Could you check a few things on this model? Use its own coordinates, in mm. Give positions to 0.01 mm unless a question says otherwise; leave off trailing zeros. Order: outer loops, then holes, each group sorted by start corner. A loop starts at its lowest first (then second) coordinate and runs counter-clockwise, first axis right, second up. Notation, with made-up numbers: M 56,69.25 L 110,69.25 A17 ccw 110,84.25 Z; hole C -36.75,25.5 d10. An arc over 180 degrees is marked long. Answer in a Markdown table with one row per item. Add a question column.
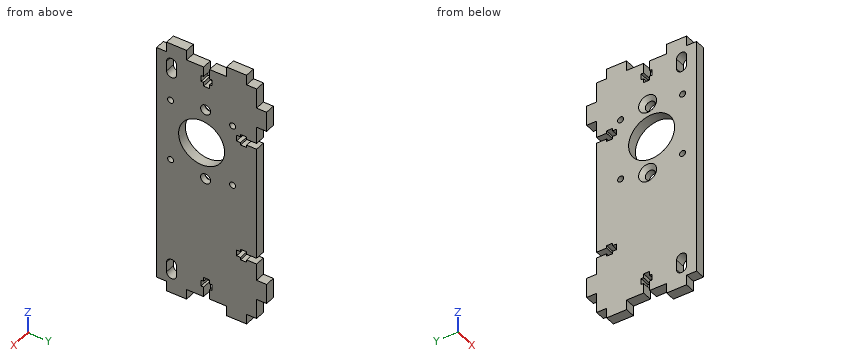
```python
from build123d import *

# Parameters (mm, degrees)
SKETCH1_W           = 120
SKETCH1_H           = 50
SKETCH1_R           = 1.5
SKETCH1_R_2         = 11.5
SKETCH1_R_3         = 2.5
BOSS_EXTRUDE1_DEPTH = 5
CHAMFER1_SIZE       = 2
SKETCH2_W           = 5
SKETCH2_H           = 10
SKETCH2_W_2         = 10
SKETCH2_H_2         = 5
BOSS_EXTRUDE2_DEPTH = 5
CUT_EXTRUDE1_DEPTH  = 137.656503687


with BuildPart() as part:
    # Sketch1 → Boss-Extrude1 (new body)
    with BuildSketch(Plane(origin=(0, 0, 0), x_dir=(0, 0, -1), z_dir=(1, 0, 0))):
        with Locations((-60, 25)):
            Rectangle(SKETCH1_W, SKETCH1_H)
        with Locations((-95.5, 38)):
            Circle(SKETCH1_R, mode=Mode.SUBTRACT)
        with Locations((-64.5, 38)):
            Circle(SKETCH1_R, mode=Mode.SUBTRACT)
        with Locations((-64.5, 7)):
            Circle(SKETCH1_R, mode=Mode.SUBTRACT)
        with Locations((-95.5, 7)):
            Circle(SKETCH1_R, mode=Mode.SUBTRACT)
        with Locations((-80, 22.5)):
            Circle(SKETCH1_R_2, mode=Mode.SUBTRACT)
        with Locations((-98, 24.5)):
            Circle(SKETCH1_R_3, mode=Mode.SUBTRACT)
        with Locations((-62, 24.5)):
            Circle(SKETCH1_R_3, mode=Mode.SUBTRACT)
    extrude(amount=BOSS_EXTRUDE1_DEPTH)

    # Chamfer1
    chamfer1_edges = [part.edges().sort_by_distance(p)[0] for p in [
        (0, 24.5, 100.5),
        (0, 24.5, 64.5),
    ]]
    chamfer(chamfer1_edges, length=CHAMFER1_SIZE)

    # Sketch2 → Boss-Extrude2 (add)
    with BuildSketch(Plane(origin=(5, 0, 0), x_dir=(0, 0, -1), z_dir=(1, 0, 0))):
        with Locations((-122.5, 10)):
            Rectangle(SKETCH2_W, SKETCH2_H)
        with Locations((-122.5, 40)):
            Rectangle(SKETCH2_W, SKETCH2_H)
        with Locations((-105, 52.5)):
            Rectangle(SKETCH2_W_2, SKETCH2_H_2)
        with Locations((-15, 52.5)):
            Rectangle(SKETCH2_W_2, SKETCH2_H_2)
        with Locations((2.5, 40)):
            Rectangle(SKETCH2_W, SKETCH2_H)
        with Locations((2.5, 10)):
            Rectangle(SKETCH2_W, SKETCH2_H)
    extrude(amount=-BOSS_EXTRUDE2_DEPTH)

    # Sketch3 → Cut-Extrude1 (cut, through all)
    with BuildSketch(Plane(origin=(5, 0, 0), x_dir=(0, 0, -1), z_dir=(1, 0, 0))):
        Polygon((0, 26.5), (-5, 26.5), (-5, 27.75), (-8, 27.75), (-8, 26.5), (-10, 26.5), (-10, 23.5), (-8, 23.5), (-8, 22.25), (-5, 22.25), (-5, 23.5), (0, 23.5), align=None)
        Polygon((-120, 23.5), (-120, 26.5), (-115, 26.5), (-115, 27.75), (-112, 27.75), (-112, 26.5), (-110, 26.5), (-110, 23.5), (-112, 23.5), (-112, 22.25), (-115, 22.25), (-115, 23.5), align=None)
        Polygon((-31.5, 50), (-31.5, 45), (-32.75, 45), (-32.75, 42), (-31.5, 42), (-31.5, 40), (-28.5, 40), (-28.5, 42), (-27.25, 42), (-27.25, 45), (-28.5, 45), (-28.5, 50), align=None)
        Polygon((-91.5, 50), (-88.5, 50), (-88.5, 45), (-87.25, 45), (-87.25, 42), (-88.5, 42), (-88.5, 40), (-91.5, 40), (-91.5, 42), (-92.75, 42), (-92.75, 45), (-91.5, 45), align=None)
        with BuildLine():
            Line((-115, 10), (-110, 10))
            ThreePointArc((-110, 10), (-107.5, 7.5), (-110, 5))
            Line((-110, 5), (-115, 5))
            ThreePointArc((-115, 5), (-117.5, 7.5), (-115, 10))
        make_face()
        with BuildLine():
            Line((-5, 10), (-10, 10))
            ThreePointArc((-10, 10), (-12.5, 7.5), (-10, 5))
            Line((-10, 5), (-5, 5))
            ThreePointArc((-5, 5), (-2.5, 7.5), (-5, 10))
        make_face()
    extrude(amount=-CUT_EXTRUDE1_DEPTH, mode=Mode.SUBTRACT)


solid = part.part
```
1. Suppose I cut it at C-C on y = 7. List the corners of the cut face in (x, z) for me, plus the area to 3 significant figures.
2. Will these pins go through, and if not, where does the flat tip stop? P1, Ø1.5, axis at x = 3.5, y = 32, coming from the +Z side; P2, Ø2.5, axis at x = 1.5, y = 53.5, coming from the +Z side; P3, Ø2.5, axis at x = 2, z = 117, coming from the +Y side.
3. Suppose I cut it at A-A on y = 38. List the corners of the cut face in (x, z) for me, plus the area to 3 significant figures.
4. If I drill on line 1 along Y through (x, z) = (3.2, 110.5); line 2 along Z through (x, y) = (1.3, 41.5); line 3 along Y through (x, z) = (3.5, 62), over which ranges is the centre line in solid material (lowest first)? Write a range as [from, to].
5. Suppose I cut it at D-D on x = 3.9. Count the separate pieces of the cut face and the enclosed holes in it, plus the area to 3 significant figures.
6. Suppose I cut it at B-B on y = 17. List the corners of the cut face in (x, z) for me, plus the area to 3 significant figures.
Findings below:
| question | item | result |
|---|---|---|
| 1 | outline | M 0,-5 L 5,-5 L 5,2.55 L 0,2.55 Z; M 0,12.45 L 5,12.45 L 5,63 L 0,63 Z; M 0,66 L 5,66 L 5,94 L 0,94 Z; M 0,97 L 5,97 L 5,107.55 L 0,107.55 Z; M 0,117.45 L 5,117.45 L 5,125 L 0,125 Z |
| 1 | area | 521 mm2 |
| 2 | P1 | z = 120 |
| 2 | P2 | z = 110 |
| 2 | P3 | y = 50 |
| 3 | outline | M 0,-5 L 5,-5 L 5,63 L 0,63 Z; M 0,66 L 5,66 L 5,94 L 0,94 Z; M 0,97 L 5,97 L 5,125 L 0,125 Z |
| 3 | area | 620 mm2 |
| 4 | line 1 | [0, 5], [10, 23.5], [26.5, 50] |
| 4 | line 2 | [-5, 28.5], [31.5, 88.5], [91.5, 125] |
| 4 | line 3 | [0, 22], [27, 50] |
| 5 | separate pieces | 1 |
| 5 | enclosed holes | 9 |
| 5 | area | 5,580 mm2 |
| 6 | outline | M 0,0 L 5,0 L 5,69.9 L 0,69.9 Z; M 0,90.1 L 5,90.1 L 5,120 L 0,120 Z |
| 6 | area | 499 mm2 |
